Part model, mm, in its own coordinate system. Face numbers are marked on the shaded views. Round coordinates to 2 decimals unless told otherwise and drop trailing zeros. Loops run counter-clockwise (first coordinate to the right, second up) from the corner with the lowest first, then second, coordinate; pieces in that order, holes last. Notation, with made-up numbers: M 18.25,16.25 L 60.25,16.25 A27 cw 60.25,54.25 Z; hole C 85,-35 d1. An arc over 180 degrees is marked long. Put each result on its own line as item: value. Start each with the question number.
1) Pull direction Z, two halves, no side cores. Call the marked faces 1, 2, 3 and 4: +Z half, -Z half, draft (parallel to the pull), parting line (faces both ways), or undercut.
2) Slice it at D-D on z = 41. Give the cut face in (x, y), then the cut area to 3 significant figures.
3) Probe line 1 along X through (y, z) = (-33, 19); line 2 along Y through (x, z) = (8.5, 45); line 3 along Z through (x, y) = (44, -14). List the from-to ranges inside material, lowest first.
4) Drop flat-ended pins along their axis: pin 1 Ø17 at (y, z) = (-19.32, 41.62) entering from -X; pin 2 Ø15 at (y, z) = (-21.5, 29) entering from +X; pin 3 Ø12 at (x, y) = (31.07, -19.29) entering from +Z; pin 4 Ø1.5 at (y, z) = (-11, 16) entering from +X. Give the stop position or say it passes through.
5) Slice it at B-B on y = -10.5. Give the cut face in (x, z).
6) Slice it at C-C on y = -21. Give the cut face in (x, z), then the cut area to 3 significant figures.
7) Slice it at A-A on x = 32.5. Give the cut face in (y, z).
```python
from build123d import *

# Parameters (mm, degrees)
F1_DEPTH  = 38.1
F3_DEPTH  = 25.4
F4_R      = 4.6186777809
F4_R_2    = 4.7220992833
F5_DEPTH  = 25.4
F7_DEPTH  = 25.4
F9_DEPTH  = 25.4
F11_DEPTH = 25.4


with BuildPart() as f1:
    # F0 (on Front) → F1 (new body)
    with BuildSketch(Plane.XZ):
        Polygon((0, 49.3678711355), (0, 0), (68.8029304147, 0), (68.8029304147, 16.7396813631), (22.272285074, 16.7396813631), (22.272285074, 49.3678711355), align=None)
    extrude(amount=F1_DEPTH)

    # F2 (on face) → F3 (cut)
    with BuildSketch(Plane.XY.offset(16.7396813631)):
        with BuildLine():
            ThreePointArc((55.7516478002, 0), (66.4469620448, -18.046107265), (60.291223228, -38.1))
            Line((60.291223228, -38.1), (68.8029304147, -38.1))
            Line((68.8029304147, -38.1), (68.8029304147, 0))
            Line((68.8029304147, 0), (55.7516478002, 0))
        make_face()
    extrude(amount=-F3_DEPTH, mode=Mode.SUBTRACT)

    # F4 (on face) → F5 (cut)
    with BuildSketch(Plane.XY.offset(16.7396813631)):
        with Locations((31.0677159578, -19.2931909114)):
            Circle(F4_R)
        with Locations((49.5097339153, -19.8606383055)):
            Circle(F4_R_2)
    extrude(amount=-F5_DEPTH, mode=Mode.SUBTRACT)

    # F6 (on face) → F7 (cut)
    with BuildSketch(Plane(origin=(0, 0, 0), x_dir=(0, -1, 0), z_dir=(-1, 0, 0))):
        with BuildLine():
            ThreePointArc((0, 37.1677689254), (19.5787852864, 48.1513039346), (38.1, 35.465426743))
            Line((38.1, 35.465426743), (38.1, 49.3678711355))
            Line((38.1, 49.3678711355), (0, 49.3678711355))
            Line((0, 49.3678711355), (0, 37.1677689254))
        make_face()
    extrude(amount=-F7_DEPTH, mode=Mode.SUBTRACT)

    # F8 (on face) → F9 (cut)
    with BuildSketch(Plane.YZ.offset(22.272285074)):
        with BuildLine():
            ThreePointArc((-11.3676669021, 46.8945718353), (-19.633075345, 48.1488087071), (-27.7434336329, 46.1209587865))
            ThreePointArc((-27.7434336329, 46.1209587865), (-18.8743086198, 32.0873075282), (-11.3676669021, 46.8945718352))
        make_face()
    extrude(amount=-F9_DEPTH, mode=Mode.SUBTRACT)

    # F10 (on face) → F11 (cut)
    with BuildSketch(Plane.XY.offset(16.7396813631)):
        with BuildLine():
            ThreePointArc((55.7516478002, 0), (62.3960801541, -18.5287656348), (60.291223228, -38.1))
            ThreePointArc((60.291223228, -38.1), (66.4469620448, -18.046107265), (55.7516478002, 0))
        make_face()
    extrude(amount=-F11_DEPTH, mode=Mode.SUBTRACT)


solid = f1.part
```
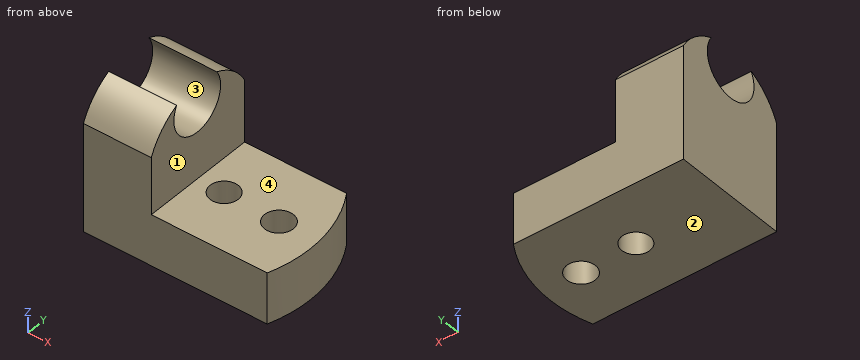
Recorded:
1. face 1: draft
1. face 2: -Z half
1. face 3: undercut
1. face 4: +Z half
2. outline: M 0,-34.56 L 22.27,-34.56 L 22.27,-28.85 L 0,-28.85 Z; M 0,-9.8 L 22.27,-9.8 L 22.27,-2.7 L 0,-2.7 Z
2. area: 285 mm2
3. line 1: x = 0 to 22.27
3. line 2: y = -29.81 to -28.25, -10.4 to -7.45
3. line 3: z = 0 to 16.74
4. pin 1: passes through
4. pin 2: stops at x = 22.27
4. pin 3: stops at z = 16.74
4. pin 4: stops at x = 61.04
5. outline: M 0,0 L 60.67,0 L 60.67,16.74 L 22.27,16.74 L 22.27,37.98 L 0,37.98 Z; M 0,45.26 L 22.27,45.26 L 22.27,46.56 L 0,46.56 Z
6. outline: M 0,0 L 26.78,0 L 26.78,16.74 L 22.27,16.74 L 22.27,32.22 L 0,32.22 Z; M 35.36,0 L 44.93,0 L 44.93,16.74 L 35.36,16.74 Z; M 54.09,0 L 62.62,0 L 62.62,16.74 L 54.09,16.74 Z
6. area: 1,100 mm2
7. outline: M -38.1,0 L -23.68,0 L -23.68,16.74 L -38.1,16.74 Z; M -14.9,0 L 0,0 L 0,16.74 L -14.9,16.74 Z
